Input: part model. Units: mm. Frame: model coordinates. Face numbers are marked on the shaded views. A direction names the side the tool comes from. Give positions to 0.01 mm unless a question says otherwise; leave off trailing zeros. Loops run counter-clockwise (first coordinate to the right, second up) from the corner with the lowest first, then second, coordinate; pieces in that order, holes last. Notation, with made-up numbers: M 8.25,-5 L 17.25,-5 A25 cw 17.25,28 Z; hole C 2.25,54.25 d1. An arc over 180 degrees is marked long. One line per item, written item: value. Start each with the question number.
(1) Access query for the marked faces 3 and 4. Directions: +Z, -Z, +X, -X, +Y, -Y. A direction counts if a zero-diameter tool reaches every point of the face in a straight line with its end or side. Return the directions, or none.
(2) Section A-A on x = -24.92. Output: boundary loops of the cut face in (y, z), plus the area to 3 significant figures.
(3) Section D-D on y = -8.5. Output: boundary loops of the cut face in (x, z).
(4) Pin query (flat end, axial travel): P1, Ø1.5, axis at x = 12.5, y = 4, coming from the -Z side; P2, Ø10, axis at x = -6, y = 7.5, coming from the +Z side; P3, Ø5, axis at x = -21, y = -1.5, coming from the +Z side. Return the tip coordinate at first contact, or that it passes through.
(5) Ray query, line 1 along Y through (x, z) = (-24.92, 0.9); line 2 along Z through (x, y) = (-24, 7.75); line 3 along X through (y, z) = (-3.5, 1.75). Return the intervals inside material, ascending. Write a range as from..to.
(6) Section C-C on z = 11. Output: boundary loops of the cut face in (x, y), plus the area to 3 significant figures.
(7) Pull-direction query (X, two-part tool) for the marked faces 1 and 2; classes: released by +X, released by -X, zero draft, split by the parting line, or undercut.
(8) Section B-B on y = 0. Output: boundary loops of the cut face in (x, z).
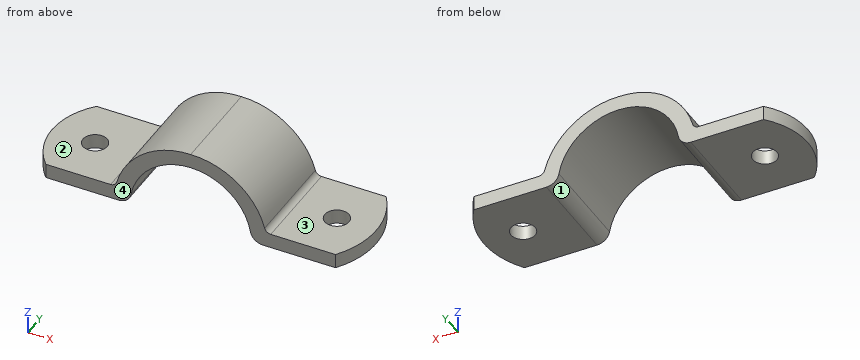
```python
from build123d import *

# Parameters (mm, degrees)
F1_DEPTH = 10
F2_R     = 2.5
F3_DEPTH = 25
F5_DEPTH = 3
F7_DEPTH = 3


with BuildPart() as f1:
    # F0 (on Front) → F1 (new body, symmetric)
    with BuildSketch(Plane.XZ):
        with BuildLine():
            ThreePointArc((-12.3133069376, 2.1523178808), (0, 12.5), (12.3133069376, 2.1523178808))
            ThreePointArc((12.3133069376, 2.1523178808), (13.2017484895, 0.6095259974), (14.8744747806, 0))
            Line((14.8744747806, 0), (29.85, 0))
            Line((29.85, 0), (29.85, 3))
            Line((29.85, 3), (16.503, 3))
            ThreePointArc((16.503, 3), (15.7100109406, 3.2698697404), (15.2462584222, 3.9674333051))
            ThreePointArc((15.2462584222, 3.9674333051), (9.6127418909, 12.3640200256), (0, 15.5))
            ThreePointArc((0, 15.5), (-9.6127418909, 12.3640200256), (-15.2462584222, 3.9674333051))
            ThreePointArc((-15.2462584222, 3.9674333051), (-15.7100109406, 3.2698697404), (-16.503, 3))
            Line((-16.503, 3), (-29.85, 3))
            Line((-29.85, 3), (-29.85, 0))
            Line((-29.85, 0), (-14.8744747806, 0))
            ThreePointArc((-14.8744747806, 0), (-13.2017484895, 0.6095259974), (-12.3133069376, 2.1523178808))
        make_face()
    extrude(amount=F1_DEPTH, both=True)

    # F2 (on face) → F3 (cut)
    with BuildSketch(Plane.XY.offset(3)):
        with Locations((24.92, 0)):
            Circle(F2_R)
        with Locations((-24.92, 0)):
            Circle(F2_R)
    extrude(amount=-F3_DEPTH, mode=Mode.SUBTRACT)

    # F4 (on face) → F5 (join)
    with BuildSketch(Plane.XY.offset(3)):
        with BuildLine():
            Line((-29.85, -10), (-29.85, 10))
            ThreePointArc((-29.85, 10), (-33.7754930507, 0), (-29.85, -10))
        make_face()
    extrude(amount=-F5_DEPTH)

    # F6 (on face) → F7 (join)
    with BuildSketch(Plane.XY.offset(3)):
        with BuildLine():
            Line((29.85, 10), (29.85, -10))
            ThreePointArc((29.85, -10), (33.0329889849, 0), (29.85, 10))
        make_face()
    extrude(amount=-F7_DEPTH)


solid = f1.part
```
Output values:
1. face 3: +Z, +X, +Y, -Y
1. face 4: +Z, -Z, +X, -X, -Y
2. outline: M -10,0 L -2.5,0 L -2.5,3 L -10,3 Z; M 2.5,0 L 10,0 L 10,3 L 2.5,3 Z
2. area: 45.0 mm²
3. outline: M -31.07,0 L -14.87,0 A2.6 ccw -12.31,2.15 A12.5 cw 12.31,2.15 A2.6 ccw 14.87,0 L 30.8,0 L 30.8,3 L 16.5,3 A1.3 cw 15.25,3.97 A15.5 ccw 0,15.5 A15.5 ccw -15.25,3.97 A1.3 cw -16.5,3 L -31.07,3 Z
4. P1: stops at z = 0.57
4. P2: stops at z = 15.48
4. P3: stops at z = 3
5. line 1: y = -10..-2.5, 2.5..10
5. line 2: z = 0..3
5. line 3: x = -33.35..-12.42, 12.42..32.68
6. outline: M -11.18,-10 L -5.94,-10 L -5.94,10 L -11.18,10 Z; M 5.94,-10 L 11.18,-10 L 11.18,10 L 5.94,10 Z
6. area: 210 mm²
7. face 1: undercut
7. face 2: zero draft
8. outline: M -33.78,0 L -27.42,0 L -27.42,3 L -33.78,3 Z; M -22.42,0 L -14.87,0 A2.6 ccw -12.31,2.15 A12.5 cw 12.31,2.15 A2.6 ccw 14.87,0 L 22.42,0 L 22.42,3 L 16.5,3 A1.3 cw 15.25,3.97 A15.5 ccw 0,15.5 A15.5 ccw -15.25,3.97 A1.3 cw -16.5,3 L -22.42,3 Z; M 27.42,0 L 33.03,0 L 33.03,3 L 27.42,3 Z
